Build history of the part. All positions in model axes, mm. A direction names the side the tool comes from. Coordinates: 2 decimals unless noted, no trailing zeros. Loops run counter-clockwise (first coordinate to the right, second up) from the corner with the lowest first, then second, coordinate; pieces in that order, holes last. Notation, with made-up numbers: (-10, 73.25) - (43, 73.25) arc R18 ccw to (43, 88.25) - close; hole circle Ø7 at (37.25, 29). An arc over 180 degrees is marked (long way). One line per item, written item: value.
Autodesk Inventor part; units mm, degrees
ref_plane "YZ Plane" through (0, 0, 0) normal (1, 0, 0) x (0, 1, 0)
ref_plane "XZ Plane" through (0, 0, 0) normal (0, 1, 0) x (-1, 0, 0)
ref_plane "XY Plane" through (0, 0, 0) normal (0, 0, 1) x (1, 0, 0)
sketch "Skizze1" plane through (0, 0, 0) normal (0, 1, 0) x (-1, 0, 0)
  line L0 (0, 0) -> (82, 0)
  line L1 (82, 0) -> (82, -99)
  line L2 (82, -99) -> (0, -99)
  line L3 (0, -99) -> (0, 0)
  dimension "d0" = 82
  dimension "d1" = 99
extrude "Extrusion1" add sketch "Skizze1" along normal blind 30
sketch "Skizze2" plane through (0, 30, 0) normal (0, 1, 0) x (1, 0, 0)
  point P0 (0, 0)
sketch "Skizze3" plane through (0, 30, 0) normal (0, 1, 0) x (1, 0, 0)
  line L0 (-82, 0) -> (0, 0)
  line L1 (0, 0) -> (0, 99)
  point P0 (-76.5, 4.5)
  point P1 (-6.5, 97)
  dimension "d4" = 4.5
  dimension "d5" = 92.5
  dimension "d7" = 6.5
  dimension "d8" = 70
hole "Bohrung1" at (-76.5, 30, -4.5) at (-6.5, 30, -97) direction (0, -1, 0) diameter 3.5 end through all
sketch "Skizze4" plane through (0, 30, 0) normal (0, 1, 0) x (1, 0, 0)
  line L0 (-82, 0) -> (0, 0)
  line L1 (-67, 0) -> (-27, 0)
  line L2 (-27, 0) -> (-27, 15)
  line L3 (-27, 15) -> (-67, 15)
  line L4 (-67, 15) -> (-67, 0)
  line L5 (-82, 99) -> (-82, 0)
  dimension "d16" = 15
  dimension "d17" = 15
  dimension "d18" = 40
extrude "Extrusion2" cut sketch "Skizze4" against normal blind 20
properties part number "PSU" material "Stahl, weich"
Item 1: Cut at A-A, the plane z = -4.5. Write the cut outline in (x, y), then the cut area to 4 significant figures.
Check result:
outline: (-82, 0) - (-78.25, 0) - (-78.25, 30) - (-82, 30) - close; (-74.75, 0) - (0, 0) - (0, 30) - (-27, 30) - (-27, 10) - (-67, 10) - (-67, 30) - (-74.75, 30) - close
area: 1,555 mm^2
Item 2: Cut at C-C, the plane y = 22.25. Write the cut outline in (x, z), then the cut area to 3 significant figures.
Check result:
outline: (-82, -99) - (0, -99) - (0, 0) - (-27, 0) - (-27, -15) - (-67, -15) - (-67, 0) - (-82, 0) - close; hole circle Ø3.5 at (-76.5, -4.5); hole circle Ø3.5 at (-6.5, -97)
area: 7,500 mm^2
Item 3: Tool access for faces 5 (the face through (0, 15, -50)), 6 (the face through (-67, 20, -8)): list every direction of +Z, -Z, +X, -X, +Y, -Y with a clear straight run to the whole face (end or side of a thin tool).
Check result:
face 5: +Z, -Z, +X, +Y, -Y
face 6: +Z, +Y
Item 4: Drop flat-ended pins along their axis: P1, Ø10, axis at x = -37.5, y = 17, coming from the +Z side; P2, Ø4.5, axis at x = -40.5, z = -7.5, coming from the +Y side; P3, Ø3, axis at x = -6.5, z = -97, coming from the -Y side. Give the stop position or say it passes through.
Check result:
P1: stops at z = -15
P2: stops at y = 10
P3: passes through
Item 5: Cut at B-B, the plane x = -76.5. Write the cut outline in (y, z), then the cut area to 4 significant figures.
Check result:
outline: (0, -99) - (30, -99) - (30, -6.25) - (0, -6.25) - close; (0, -2.75) - (30, -2.75) - (30, 0) - (0, 0) - close
area: 2,865 mm^2
Item 6: Pull direction Z, two halves, no side cores. Call faces 1 (the face through (-47, 20, -15)), 2 (the face through (-40, 30, -49)), 3 (the face through (-42, 15, -99)), 4 (the face through (-4.79, 14.79, -97.38)): released by +Z, released by -Z, zero draft, split by the parting line, or undercut.
Check result:
face 1: released by +Z
face 2: zero draft
face 3: released by -Z
face 4: undercut
Item 7: Cut at D-D, the plane z = -97. Write the cut outline in (x, y), then the cut area to 4 significant figures.
Check result:
outline: (-82, 0) - (-8.25, 0) - (-8.25, 30) - (-82, 30) - close; (-4.75, 0) - (0, 0) - (0, 30) - (-4.75, 30) - close
area: 2,355 mm^2
Item 8: Probe probe 1 along X at (y, z) = (12, -4.5); probe 2 along X at (y, z) = (11.5, -97); probe 3 along Z at (x, y) = (-76.5, 8). List the from-to ranges inside material, lowest first. Write a range as from..to.
Check result:
probe 1: x = -82..-78.25, -74.75..-67, -27..0
probe 2: x = -82..-8.25, -4.75..0
probe 3: z = -99..-6.25, -2.75..0
